Answer from the drawing. Dimensions are ordinates in mm from the lowest x, y and z of the part. A direction names the side the tool comes from. Round coordinates to 2 decimals unless told otherwise and drop trailing zeros. Write each loop counter-clockwise with the first axis right and the second up, starting at its lowest first coordinate (ties: lowest second). Pieces come first, ordered by that corner, then holes. Notation, with made-up numbers: M 89.5,31.25 L 102.5,31.25 A15 cw 102.5,46.25 Z; hole C 21.25,81.5 d4. An arc over 180 degrees is marked long. One line per item, written item: value. Start each with the question number.
(1) Section C-C (z = 16) is taken. Determine the outline of the cut face in (x, y).
(2) Given P1, Ø3, axis at x = 27, y = 19.5, coming from the -Z side; P2, Ø9.5, axis at y = 27, z = 28, coming from the -X side; P3, Ø4, axis at x = 49.5, z = 57, coming from the -Y side, each flat-ended and moving along its own axis, determine where each tip first touches the part or whether it passes through.
(3) Section A-A (y = 20) is taken. Determine the outline of the cut face in (x, z).
(4) For the marked faces 4 and 5, determine the directions among +Z, -Z, +X, -X, +Y, -Y from which every point of the face is accessible in a straight line to the end or side of a thin tool.
(5) For a pull along X with two mould halves and no side action, classify the marked faces 1, 2 and 3 as released by +X, released by -X, zero draft, split by the parting line, or undercut.
(6) Section B-B (x = 43.5) is taken. Determine the outline of the cut face in (y, z).
(7) Consider probe 1 along X at (y, z) = (10.5, 31); probe 2 along X at (y, z) = (27, 31.5); probe 3 along Y at (x, z) = (35, 37). Determine where each line is inside the solid, lowest interval first.
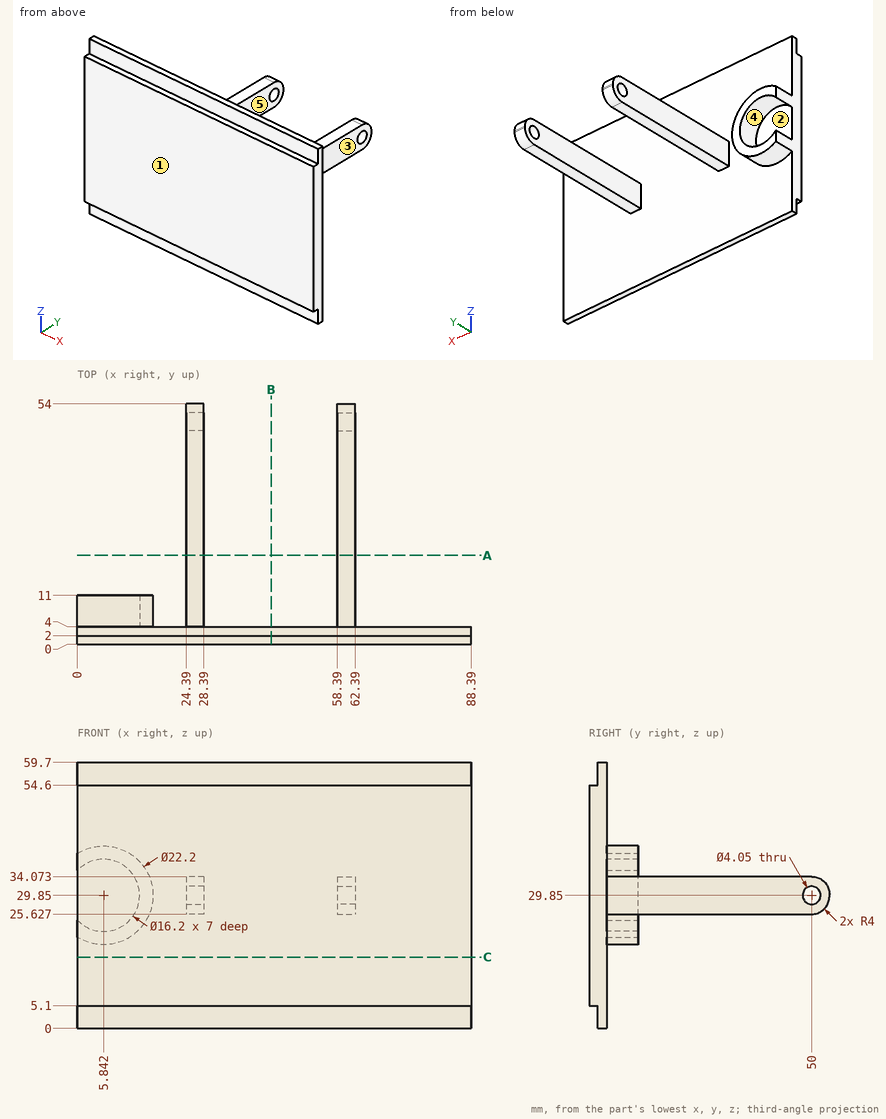
Recorded:
1. outline: M 0,0 L 88.39,0 L 88.39,4 L 0,4 Z
2. P1: stops at z = 25.63
2. P2: stops at x = 24.39
2. P3: stops at y = 2
3. outline: M 24.39,25.63 L 28.39,25.63 L 28.39,34.07 L 24.39,34.07 Z; M 58.39,25.63 L 62.39,25.63 L 62.39,34.07 L 58.39,34.07 Z
4. face 4: +Y
4. face 5: +Z, -Z, +Y
5. face 1: zero draft
5. face 2: undercut
5. face 3: released by +X
6. outline: M 0,5.1 L 2,5.1 L 2,0 L 4,0 L 4,59.7 L 2,59.7 L 2,54.6 L 0,54.6 Z
7. probe 1: x = 13.86 to 16.88, 24.39 to 28.39, 58.39 to 62.39
7. probe 2: x = 24.39 to 28.39, 58.39 to 62.39
7. probe 3: y = 0 to 4
